```python
from build123d import *

# Parameters (mm, degrees)
SKETCH1_W                                           = 81.999999998
SKETCH1_H                                           = 60
BOSS_EXTRUDE1_DEPTH                                 = 19
TAP_DRILL_FOR_M6_TAP1_D                             = 5
CSK_FOR_M6_COUNTERSUNK_FLAT_HEAD_SCREW1_D           = 6.6
CSK_FOR_M6_COUNTERSUNK_FLAT_HEAD_SCREW1_CSINK_D     = 12.6
CSK_FOR_M6_COUNTERSUNK_FLAT_HEAD_SCREW1_CSINK_ANGLE = 90
SKETCH7_W                                           = 81.999999998
SKETCH7_H                                           = 4
CUT_EXTRUDE1_DEPTH                                  = 20
SKETCH10_W                                          = 81.999999998
SKETCH10_H                                          = 0.95
BOSS_EXTRUDE2_DEPTH                                 = 19
FILLET1_R                                           = 4
TAP_DRILL_FOR_M5_TAP1_D                             = 4.2
TAP_DRILL_FOR_M5_TAP1_DEPTH                         = 30
TAP_DRILL_FOR_M5_TAP1_TIP                           = 1.2618073
TAP_DRILL_FOR_M5_TAP2_D                             = 4.2


with BuildPart() as part:
    # Sketch1 → Boss-Extrude1 (new body)
    with BuildSketch(Plane.XY):
        with Locations((20.999999999, 38.745248777)):
            Rectangle(SKETCH1_W, SKETCH1_H)
    extrude(amount=BOSS_EXTRUDE1_DEPTH)

    # Tap Drill for M6 Tap1 (through all)
    with Locations(Plane.XY.offset(19)):
        with Locations((8.999999998, 58.745248777), (54.999999998, 58.745248777), (54.999999998, 45.745248777), (8.999999998, 45.745248777)):
            Hole(TAP_DRILL_FOR_M6_TAP1_D / 2)

    # CSK for M6 Countersunk Flat Head Screw1 (through all)
    with Locations(Plane(origin=(0, 0, 0), x_dir=(1, 0, 0), z_dir=(0, 0, -1))):
        with Locations((0, -21.745248777), (0, -52.745248777)):
            CounterSinkHole(CSK_FOR_M6_COUNTERSUNK_FLAT_HEAD_SCREW1_D / 2, CSK_FOR_M6_COUNTERSUNK_FLAT_HEAD_SCREW1_CSINK_D / 2, counter_sink_angle=CSK_FOR_M6_COUNTERSUNK_FLAT_HEAD_SCREW1_CSINK_ANGLE)

    # Sketch7 → Cut-Extrude1 (cut, through all)
    with BuildSketch(Plane(origin=(0, 0, 0), x_dir=(-1, 0, 0), z_dir=(0, 0, -1))):
        with Locations((-20.999999999, 66.745248777)):
            Rectangle(SKETCH7_W, SKETCH7_H)
    extrude(amount=-CUT_EXTRUDE1_DEPTH, mode=Mode.SUBTRACT)

    # Sketch10 → Boss-Extrude2 (add)
    with BuildSketch(Plane(origin=(0, 0, 0), x_dir=(-1, 0, 0), z_dir=(0, 0, -1))):
        with Locations((-20.999999999, 8.270248777)):
            Rectangle(SKETCH10_W, SKETCH10_H)
    extrude(amount=-BOSS_EXTRUDE2_DEPTH)

    # Fillet1
    fillet1_edges = [part.edges().sort_by_distance(p)[0] for p in [
        (-20, 64.745248777, 9.5),
        (61.999999998, 64.745248777, 9.5),
        (61.999999998, 7.795248777, 9.5),
        (-20, 7.795248777, 9.5),
    ]]
    fillet(fillet1_edges, radius=FILLET1_R)

    # Tap Drill for M5 Tap1
    with Locations(Plane(origin=(0, 7.795248777, 0), x_dir=(-1, 0, 0), z_dir=(0, -1, 0))):
        with Locations((-41.999999998, -9.499999998)):
            Hole(TAP_DRILL_FOR_M5_TAP1_D / 2, depth=TAP_DRILL_FOR_M5_TAP1_DEPTH)
            with Locations((0, 0, -(TAP_DRILL_FOR_M5_TAP1_DEPTH + TAP_DRILL_FOR_M5_TAP1_TIP / 2))):  # 118° drill point
                Cone(0, TAP_DRILL_FOR_M5_TAP1_D / 2, TAP_DRILL_FOR_M5_TAP1_TIP, mode=Mode.SUBTRACT)

    # Tap Drill for M5 Tap2 (through all)
    with Locations(Plane.XY.offset(19)):
        with Locations((54.999999998, 35.395248777), (54.999999998, 48.395248777), (8.999999998, 35.395248777), (8.999999998, 48.395248777)):
            Hole(TAP_DRILL_FOR_M5_TAP2_D / 2)


solid = part.part
```
Can you work these out from the model? Positions are in its coordinate system, mm. A direction names the side the tool comes from. Give positions to 0.01 mm unless a question says otherwise; leave off trailing zeros. Order: outer loops, then holes, each group sorted by start corner. A loop starts at its lowest first (then second) coordinate and runs counter-clockwise, first axis right, second up. Notation, with made-up numbers: M 8.25,-35.75 L 42.25,-35.75 A9 ccw 42.25,-23.75 Z; hole C 37,33.5 d4. An arc over 180 degrees is marked long. Write item = value, one per line. Start each with the question number.
Q1. Will these pins go through, and if not, where does the flat tip stop? pin 1 Ø10.5 at (x, y) = (0, 21.75) entering from -Z; pin 2 Ø7.5 at (x, y) = (0, 52.75) entering from -Z; pin 3 Ø4 at (x, y) = (9, 58.75) entering from +Z.
Q2. Suppose I cut it at C-C (z = 14). Count the separate pieces of the cut face and the enclosed holes in it, plus the area to 3 significant figures.
Q3. Suppose I cut it at B-B (x = 0). Write out the boundary of the cut face in (y, z), plus the area to 3 significant figures.
Q4. I need wall thicknesses on probe 1 along Y at (x, z) = (55, 13.25); probe 2 along X at (y, z) = (48.5, 13); probe 3 along Y at (x, z) = (0.5, 10.25). Which ranges of each line are inside material? Lowest first, please. Write a range as [from, to].
Q5. We'd pull the mould along X, two halves only. Please class faces 1 (the flat face through (22, 64.745, 9)), 2 (the flat face through (-20, 36, 9)), 3 (the cylindrical face through (9.081, 43.247, 9.367)): pulls with the +X half, pulls with the -X half, needs draft (parallel to the pull), parting line crosses it, or undercut.
Q6. For faces 4 (the cylindrical face through (2.43, 19.51, 11.11)), 5 (the cylindrical face through (42.969, 23.005, 11.363)), which set-ups out of +Z, -Z, +X, -X, +Y, -Y let a thin tool reach every point of the face, with its end or its side?
Q7. Suppose I cut it at A-A (x = 55). Write out the boundary of the cut face in (y, z).
Check result:
q1.pin_1 = 1.05
q1.pin_2 = 2.55
q1.pin_3 = through
q2.separate_pieces = 1
q2.enclosed_holes = 8
q2.area = 4,460 mm2
q3.outline = M 7.8,0 L 15.45,0 L 18.45,3 L 18.45,19 L 7.8,19 Z; M 25.05,3 L 28.05,0 L 46.45,0 L 49.45,3 L 49.45,19 L 25.05,19 Z; M 56.05,3 L 59.05,0 L 64.75,0 L 64.75,19 L 56.05,19 Z
q3.area = 813 mm2
q4.probe_1 = [7.8, 33.3], [37.5, 43.25], [50.5, 56.25], [61.25, 64.75]
q4.probe_2 = [-20, 6.9], [11.1, 52.9], [57.1, 62]
q4.probe_3 = [7.8, 18.48], [25.01, 49.48], [56.01, 64.75]
q5.face_1 = needs draft
q5.face_2 = pulls with the -X half
q5.face_3 = undercut
q6.face_4 = +Z, -Z
q6.face_5 = -Y
q7.outline = M 7.8,0 L 33.3,0 L 33.3,19 L 7.8,19 Z; M 37.5,0 L 43.25,0 L 43.25,19 L 37.5,19 Z; M 50.5,0 L 56.25,0 L 56.25,19 L 50.5,19 Z; M 61.25,0 L 64.75,0 L 64.75,19 L 61.25,19 Z
